Read the model definition and answer for the solid it produces. Units are mm, in the model's axes. Face numbers are marked on the shaded views. A direction names the side the tool comes from. Round coordinates to 2 decimals unless told otherwise and drop trailing zeros. Loops run counter-clockwise (first coordinate to the right, second up) from the corner with the lowest first, then second, coordinate; pieces in that order, holes last. Notation, with made-up numbers: M -11.5,-31.75 L 23.5,-31.75 A23 ccw 23.5,-19.75 Z; hole C 61,24.25 d11. An arc over 180 degrees is marked long. Write each question's results on one line, items separated by ' | '.
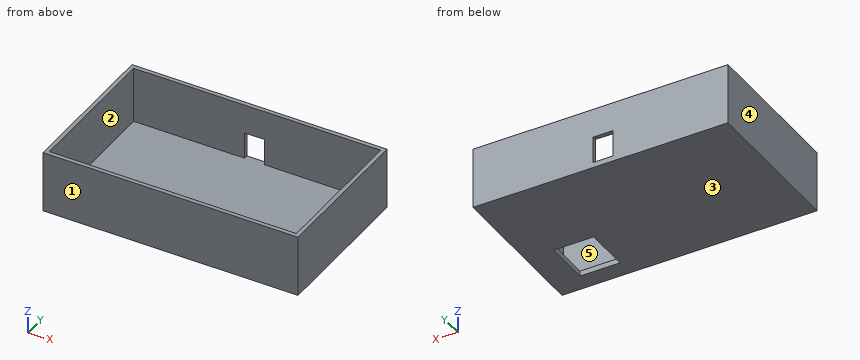
from build123d import *

# Parameters (mm, degrees)
F0_W     = 95.5
F0_H     = 57.5
F0_W_2   = 92.5
F0_H_2   = 54.5
F0_W_3   = 90.5
F0_H_3   = 52.5
F1_DEPTH = 2
F2_DEPTH = 21
F3_W     = 7.5
F3_H     = 10
F4_DEPTH = 1.5
F5_W     = 15
F5_H     = 17
F6_DEPTH = 2
F7_ANGLE = 180


with BuildPart() as f1:
    # F0 (on Top) → F1 (new body)
    with BuildSketch(Plane.XY):
        with Locations((46.25, -27.25)):
            Rectangle(F0_W, F0_H)
        with Locations((46.25, -27.25)):
            Rectangle(F0_W_2, F0_H_2, mode=Mode.SUBTRACT)
        with Locations((46.25, -27.25)):
            Rectangle(F0_W_2, F0_H_2)
        with Locations((46.25, -27.25)):
            Rectangle(F0_W_3, F0_H_3, mode=Mode.SUBTRACT)
        with Locations((46.25, -27.25)):
            Rectangle(F0_W_3, F0_H_3)
    extrude(amount=F1_DEPTH)

    # F0 (on Top) → F2 (join)
    with BuildSketch(Plane.XY):
        with Locations((46.25, -27.25)):
            Rectangle(F0_W, F0_H)
        with Locations((46.25, -27.25)):
            Rectangle(F0_W_2, F0_H_2, mode=Mode.SUBTRACT)
    extrude(amount=-F2_DEPTH)

    # F3 (on face) → F4 (cut, through all)
    with BuildSketch(Plane(origin=(0, -54.5, 0), x_dir=(-1, 0, 0), z_dir=(0, 1, 0))):
        with Locations((-45.25, -5)):
            Rectangle(F3_W, F3_H)
    extrude(amount=-F4_DEPTH, mode=Mode.SUBTRACT)

    # F5 (on face) → F6 (cut, through all)
    with BuildSketch(Plane(origin=(0, 0, 0), x_dir=(1, 0, 0), z_dir=(0, 0, -1))):
        with Locations((76, 13.5)):
            Rectangle(F5_W, F5_H)
    extrude(amount=-F6_DEPTH, mode=Mode.SUBTRACT)


with BuildPart() as f1_1:
    # F7: moved
    add(f1.part.rotate(Axis((46.25, 1.5, -21), (1, 0, 0)), F7_ANGLE))


solid = f1_1.part
Item 1: Straight lines are drawn through the part: line 1 (X direction, y = 44.5, z = -25.75); line 2 (Y direction, x = 14, z = -23); line 3 (Z direction, x = 46, y = 30). For each, find the intervals that lie inside material, in ascending order.
Outcome:
line 1: x = -1.5 to 0, 92.5 to 94 | line 2: y = 1.5 to 3, 57.5 to 59 | line 3: z = -44 to -42
Item 2: The part is cut by section D-D (z = -31). Determine the outline of the cut face in (x, y).
Outcome:
outline: M -1.5,1.5 L 94,1.5 L 94,59 L -1.5,59 Z; hole M 0,3 L 92.5,3 L 92.5,57.5 L 0,57.5 Z
Item 3: The mould has two halves that part along X. Classify the marked faces 3, 4 and 5: pulls with the +X half, pulls with the -X half, needs draft (parallel to the pull), parting line crosses it, or undercut.
Outcome:
face 3: needs draft | face 4: pulls with the -X half | face 5: undercut
Item 4: The part is cut by section B-B (x = 75). Determine the outline of the cut face in (y, z), plus the area to 3 significant figures.
Outcome:
outline: M 1.5,-44 L 8,-44 L 8,-42 L 3,-42 L 3,-21 L 1.5,-21 Z; M 25,-44 L 59,-44 L 59,-21 L 57.5,-21 L 57.5,-42 L 25,-42 Z | area: 144 mm2
Item 5: The part is cut by section C-C (y = 50.5). Determine the outline of the cut face in (x, z), plus the area to 3 significant figures.
Outcome:
outline: M -1.5,-44 L 94,-44 L 94,-21 L 92.5,-21 L 92.5,-42 L 0,-42 L 0,-21 L -1.5,-21 Z | area: 254 mm2
Item 6: For the marked faces 1 and 2, determine the directions among +Z, -Z, +X, -X, +Y, -Y from which every point of the face is accessible in a straight line to the end or side of a thin tool.
Outcome:
face 1: +Z, -Z, +X, -X, -Y | face 2: +Z
Item 7: The part is cut by section A-A (y = 22). Determine the outline of the cut face in (x, z), plus the area to 3 significant figures.
Outcome:
outline: M -1.5,-44 L 68.5,-44 L 68.5,-42 L 0,-42 L 0,-21 L -1.5,-21 Z; M 83.5,-44 L 94,-44 L 94,-21 L 92.5,-21 L 92.5,-42 L 83.5,-42 Z | area: 224 mm2
Item 8: A flat-ended cylindrical pin translates along its axis: pin 1 (1.5 mm diameter, centred on x = 43.5, y = 39, fed in from +Z). Find the tip coordinate at first contact, or state that the pin passes through.
Outcome:
pin 1: stops at z = -42
